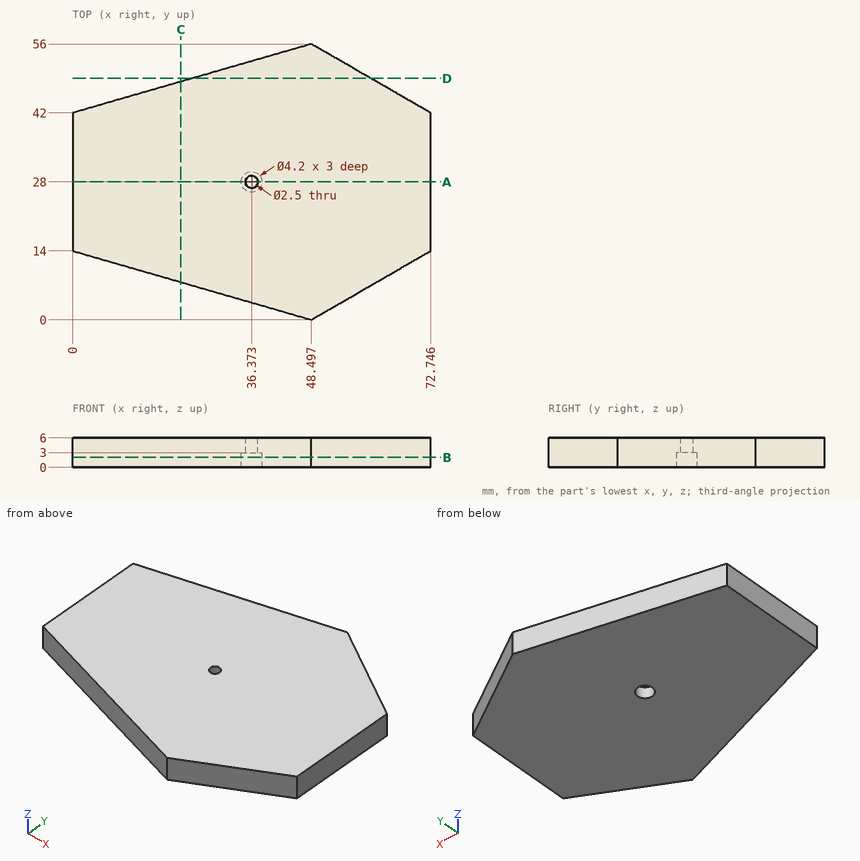
Design review of the part shown in the three views and the two pictorial views. Dimensions are in mm from the part's minimum x, y and z. Coordinates: 2 decimals unless noted, no trailing zeros. Loops run counter-clockwise (first coordinate to the right, second up) from the corner with the lowest first, then second, coordinate; pieces in that order, holes last.
(1) Consider section C-C, the plane x = 22. Give the boundary of the cut face in (y, z), plus the area to 3 significant figures.
Determined:
outline: (7.65, 0) - (48.35, 0) - (48.35, 6) - (7.65, 6) - close
area: 244 mm2
(2) Consider section B-B, the plane z = 2. Give the boundary of the cut face in (x, y), plus the area to 3 significant figures.
Determined:
outline: (0, 14) - (48.5, 0) - (72.75, 14) - (72.75, 42) - (48.5, 56) - (0, 42) - close; hole circle Ø4.2 at (36.37, 28)
area: 3,040 mm2
(3) Consider section A-A, the plane y = 28. Give the boundary of the cut face in (x, z).
Determined:
outline: (0, 0) - (34.27, 0) - (34.27, 3) - (35.12, 3) - (35.12, 6) - (0, 6) - close; (37.62, 3) - (38.47, 3) - (38.47, 0) - (72.75, 0) - (72.75, 6) - (37.62, 6) - close
(4) Consider section D-D, the plane y = 49. Give the boundary of the cut face in (x, z), plus the area to 3 significant figures.
Determined:
outline: (24.25, 0) - (60.62, 0) - (60.62, 6) - (24.25, 6) - close
area: 218 mm2
(5) Wall thickness on L1, parallel to Y at x = 46, z = 4; L2, parallel to Y at x = 26, z = 1.6 (1 decimal): over which ranges is each line inside the solid? List them lowest first.
Determined:
L1: y = 0.72 to 55.28
L2: y = 6.5 to 49.5
(6) Insertion check: P1, Ø1, axis at x = 18, z = 1, coming from the -Y side; P2, Ø1.5, axis at x = 64.5, z = 3, coming from the +Y side (1 decimal). Each pin has a flat end and moves straight along its axis. Give the tip position at first contact, or say it passes through.
Determined:
P1: stops at y = 8.66
P2: stops at y = 47.2
